Autodesk Inventor part; units mm, degrees
ref_plane "Work Plane1" through (0, 0, 3) normal (0, 0, 1) x (1, 0, 0)
ref_plane "YZ Plane" through (0, 0, 0) normal (1, 0, 0) x (0, 1, 0)
ref_plane "XZ Plane" through (0, 0, 0) normal (0, 1, 0) x (-1, 0, 0)
sketch "Sketch1" plane through (0, 0, 0) normal (0, 0, 1) x (1, 0, 0)
  line L0 (0, 0) -> (0, 45)
  line L1 (0, 0) -> (14.1421, 14.1421)
  line L2 (0, 0) -> (20, 0) construction
  line L3 (14.1421, 14.1421) -> (0, 14.1421)
  circle A0 centre (0, 0) radius 1
  circle A1 centre (14.1421, 14.1421) radius 1
  circle A2 centre (0, 45) radius 1
  circle A3 centre (0, 0) radius 2.25
  circle A4 centre (0, 45) radius 2.25
  dimension "d0" = 45
  dimension "d1" = 20
  dimension "d2" = 45
  dimension "d3" = 2
  dimension "d4" = 2
  dimension "d5" = 2
  dimension "d6" = 4.5
  dimension "d10" = 4.5
ref_plane "Work Plane1" through (0, 0, 3) normal (0, 0, 1) x (1, 0, 0)
sketch "Sketch2" plane through (0, 0, 3) normal (0, 0, 1) x (1, 0, 0)
  circle A0 centre (0, 0) radius 1
  circle A1 centre (0, 0) radius 2.25
  circle A2 centre (14.1421, 14.1421) radius 1
  circle A3 centre (0, 45) radius 1
  circle A4 centre (0, 45) radius 2.25
  line L0 (0, 0) -> (0, 45)
extrude "Extrusion1" add sketch "Sketch2" along normal blind 1.5 contours A1
sketch "Sketch3" plane through (0, 0, 3) normal (0, 0, 1) x (1, 0, 0)
  point P0 (0, 0)
extrude "Extrusion2" add sketch "Sketch2" along normal blind 1.5 contours A4
sketch "Sketch4" plane through (0, 0, 3) normal (0, 0, 1) x (1, 0, 0)
  circle A0 centre (0, 0) radius 2.25
  line L0 (-2.25, 0) -> (-2.25, 45)
  circle A1 centre (0, 45) radius 2.25
  line L1 (2.25, 45) -> (9.3211, 37.9289)
  line L2 (2.25, 45) -> (12.25, 45) construction
  line L3 (9.3211, 37.9289) -> (9.3211, 22.9289)
  dimension "d13" = 10
  dimension "d14" = 45
  dimension "d15" = 15
sketch "Sketch5" plane through (0, 0, 3) normal (0, 0, 1) x (1, 0, 0)
  circle A0 centre (14.1421, 14.1421) radius 1
  circle A1 centre (14.1421, 14.1421) radius 2
  point P0 (0, 0)
  dimension "d16" = 4
extrude "Extrusion3" add sketch "Sketch5" along normal blind 1.5
sketch "Sketch6" plane through (0, 0, 3) normal (0, 0, 1) x (1, 0, 0)
  circle A0 centre (0, 45) radius 2.25
  line L0 (2.25, 45) -> (9.3211, 37.9289)
  line L1 (2.25, 45) -> (12.25, 45) construction
  line L2 (9.3211, 37.9289) -> (9.3211, 22.9289)
  line L3 (9.3211, 22.9289) -> (15.6683, 15.4347)
  circle A1 centre (14.1421, 14.1421) radius 2
  line L4 (-2.25, 45) -> (-2.25, 0)
  circle A2 centre (0, 0) radius 2.25
  circle A3 centre (14.1421, 14.1421) radius 2
  circle A4 centre (14.1421, 14.1421) radius 1
  line L5 (2.25, 0) -> (14.4102, 12.1602)
  line L6 (2.25, 0) -> (19.4471, 0) construction
  arc A5 (-2.25, 45) -> (2.25, 45) centre (0, 45) ccw
  line L7 (2.25, 45) -> (9.3211, 37.9289)
  line L8 (9.3211, 22.9289) -> (9.3211, 37.9289)
  line L9 (9.3211, 22.9289) -> (15.6683, 15.4347)
  line L10 (14.4102, 12.1602) -> (2.25, 0)
  circle A6 centre (14.1421, 14.1421) radius 2
  circle A7 centre (0, 0) radius 2.25
  line L11 (-2.25, 0) -> (-2.25, 45)
  circle A8 centre (0, 45) radius 2.25
  arc A9 (-2.25, 45) -> (2.25, 45) centre (0, 45) ccw
  arc A10 (15.6683, 15.4347) -> (14.4102, 12.1602) centre (14.1421, 14.1421) ccw
  arc A11 (2.25, 0) -> (-2.25, 0) centre (0, 0) ccw
  dimension "d19" = 10
  dimension "d20" = 45
  dimension "d21" = 15
  dimension "d22" = 45
extrude "Extrusion4" add sketch "Sketch6" along normal blind 2.5 contours L0 L2 L3 A1 L5 A2 L4 A0
mirror "Mirror1" about plane through (0, 0, 0) normal (0, 0, 1) of "Extrusion4"
mirror "Mirror2" about plane through (0, 0, 0) normal (0, 0, 1) of "Extrusion2", "Extrusion3", "Extrusion1"
sketch "Sketch7" plane through (-2.25, 0, -5.5) normal (-1, 0, 0) x (0, 0, 1)
  point P0 (5.5, 0)
sketch "Sketch9" plane through (9.3211, 22.9289, -3) normal (1, 0, 0) x (0, 0, -1)
  line L0 (-6, 13.0711) -> (0, 13.0711)
  line L1 (0, 13.0711) -> (0, 0)
  line L2 (0, 0) -> (-6, 0)
  line L3 (-6, 0) -> (-6, 13.0711)
  point P0 (-3, -22.9289)
extrude "Extrusion6" add sketch "Sketch9" against normal blind 2
sketch "Sketch12" plane through (9.3211, 22.9289, 5.5) normal (1, 0, 0) x (0, 0, -1)
  line L0 (8.5, 13.0711) -> (2.5, 13.0711)
  line L1 (6.5, 7.0711) -> (6.5, -16.9289)
  line L2 (4.5, 13.0711) -> (6.5, 13.0711)
  line L3 (6.5, 13.0711) -> (6.5, 6.5711)
  line L4 (6.5, 6.5711) -> (4.5, 6.5711)
  line L5 (4.5, 6.5711) -> (4.5, 13.0711)
  point P0 (5.5, -22.9289)
  point P1 (5.5, 13.0711)
  dimension "d50" = 6.5
extrude "Extrusion9" cut sketch "Sketch12" against normal blind 3
sketch "Sketch14" plane through (-2.25, 0, 3) normal (-1, 0, 0) x (0, 0, 1)
  line L0 (0, 45) -> (0, 0)
  line L1 (-6, 45) -> (-6, 0)
  line L2 (-6, 2.25) -> (0, 2.25)
  line L3 (-7.5, 0) -> (-7.5, 2.25)
  line L4 (-6, 2.25) -> (-6, 7.25)
  line L5 (-6, 7.25) -> (0, 7.25)
  line L6 (0, 0) -> (0, 12.1602)
  line L7 (-6, 4.75) -> (0, 4.75)
  line L8 (-2, 2.25) -> (-4, 2.25)
  line L9 (-4, 2.25) -> (-4, 4.75)
  line L10 (-4, 4.75) -> (-2, 4.75)
  line L11 (-2, 4.75) -> (-2, 2.25)
  line L12 (-6, 7.25) -> (0, 7.25)
  line L13 (0, 7.25) -> (0, 4.75)
  line L14 (0, 4.75) -> (-6, 4.75)
  line L15 (-6, 4.75) -> (-6, 7.25)
  line L16 (-4, 4.75) -> (-2, 4.75)
  line L17 (-2, 4.75) -> (-2, 2.25)
  line L18 (-2, 2.25) -> (-4, 2.25)
  line L19 (-4, 2.25) -> (-4, 4.75)
  point P0 (-3, 0)
  point P1 (-3, 2.25)
  dimension "d53" = 5
  dimension "d54" = 2
extrude "Extrusion10" add sketch "Sketch14" against normal blind 2 contours L0 L7 L1 L5 | L11 L2 L9 L7
ref_plane "Work Plane2" through (0, 0, 0) normal (0, 0, 1) x (1, 0, 0)
properties part number "Finger_Lower_main_1"
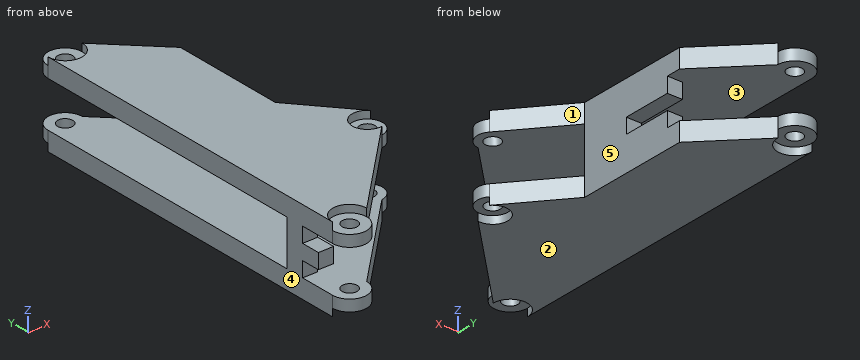
Geometry check sheet. Reference: the model listing, model coordinates, mm. Face numbers are marked on the shaded views. A direction names the side the tool comes from. Give positions to 0.01 mm unless a question says otherwise; leave off trailing zeros. Loops run counter-clockwise (first coordinate to the right, second up) from the corner with the lowest first, then second, coordinate; pieces in that order, holes last. Notation, with made-up numbers: M -31,59.25 L -17,59.25 A17 cw -17,67.25 Z; hole C -31,51 d8. An arc over 180 degrees is marked long. Write item = value, one per line. Start each with the question number.
1. Section check B-B, the plane z = -1.5. Enter the section's corners in (x, y), plus the area to 3 significant figures.
2. Section check C-C, the plane y = 35. Enter the section's corners in (x, z), plus the area to 3 significant figures.
3. Go/stop test with flat-tipped pins: P1, Ø0.6, axis at x = 8, z = 0, coming from the -Y side; P2, Ø1.6, axis at x = -1, z = 0, coming from the -Y side; P3, Ø3, axis at x = 4.5, z = -4, coming from the +Y side. Record where each tip stops, or that it passes through.
4. Thickness scan on probe 1 along Z at (x, y) = (1, 15.5); probe 2 along X at (y, z) = (45, 3.7); probe 3 along X at (y, z) = (25.5, 1). Record the ranges inside material, lowest first.
5. Section check A-A, the plane x = 3.5. Enter the section's corners in (y, z), plus the area to 4 significant figures.
6. Draft check along Z on the marked faces 1, 2 and 3. Enter one of: +Z half, -Z half, draft (parallel to the pull), parting line (faces both ways), or undercut.
7. Section check D-D, the plane z = -3.75. Enter the section's corners in (x, y), plus the area to 3 significant figures.
8. Tool access check on the marked faces 4 and 5. Record the directions out of +Z, -Z, +X, -X, +Y, -Y that give a thin tool (end or side, any length) a straight path to the whole face; none if there is none.
Values follow:
q1.outline = M -2.25,4.75 L -0.25,4.75 L -0.25,7.25 L -2.25,7.25 Z; M 7.32,22.93 L 9.32,22.93 L 9.32,36 L 7.32,36 Z
q1.area = 31.1 mm^2
q2.outline = M -2.25,-5.5 L 9.32,-5.5 L 9.32,-1 L 7.32,-1 L 7.32,-3 L -2.25,-3 Z; M -2.25,3 L 7.32,3 L 7.32,1 L 9.32,1 L 9.32,5.5 L -2.25,5.5 Z
q2.area = 65.9 mm^2
q3.P1 = 22.93
q3.P2 = 2.25
q3.P3 = 44.25
q4.probe_1 = -5.5 to -3, 3 to 5.5
q4.probe_2 = -2.25 to -1, 1 to 2.25
q4.probe_3 = 7.32 to 9.32
q5.outline = M 1.25,-5.5 L 43.75,-5.5 L 43.75,-3 L 1.25,-3 Z; M 1.25,3 L 43.75,3 L 43.75,5.5 L 1.25,5.5 Z
q5.area = 212.5 mm^2
q6.face_1 = draft
q6.face_2 = -Z half
q6.face_3 = undercut
q7.outline = M -2.25,0 A2.25 ccw 2.25,0 L 14.41,12.16 A2 ccw 15.67,15.43 L 9.32,22.93 L 9.32,37.93 L 2.25,45 A2.25 ccw -2.25,45 Z; hole C 0,0 d2; hole C 0,45 d2; hole C 14.14,14.14 d2
q7.area = 535 mm^2
q8.face_4 = +Z, -Z, -X, +Y, -Y
q8.face_5 = +Z, -Z, +X, +Y
